The drawing under review shows one solid part. Ordinate dimensions are in mm from its lowest x, y, z. A direction names the side the tool comes from. Coordinates: 2 decimals unless noted, no trailing zeros. Order: outer loops, then holes, each group sorted by start corner. A loop starts at its lowest first (then second) coordinate and runs counter-clockwise, first axis right, second up.
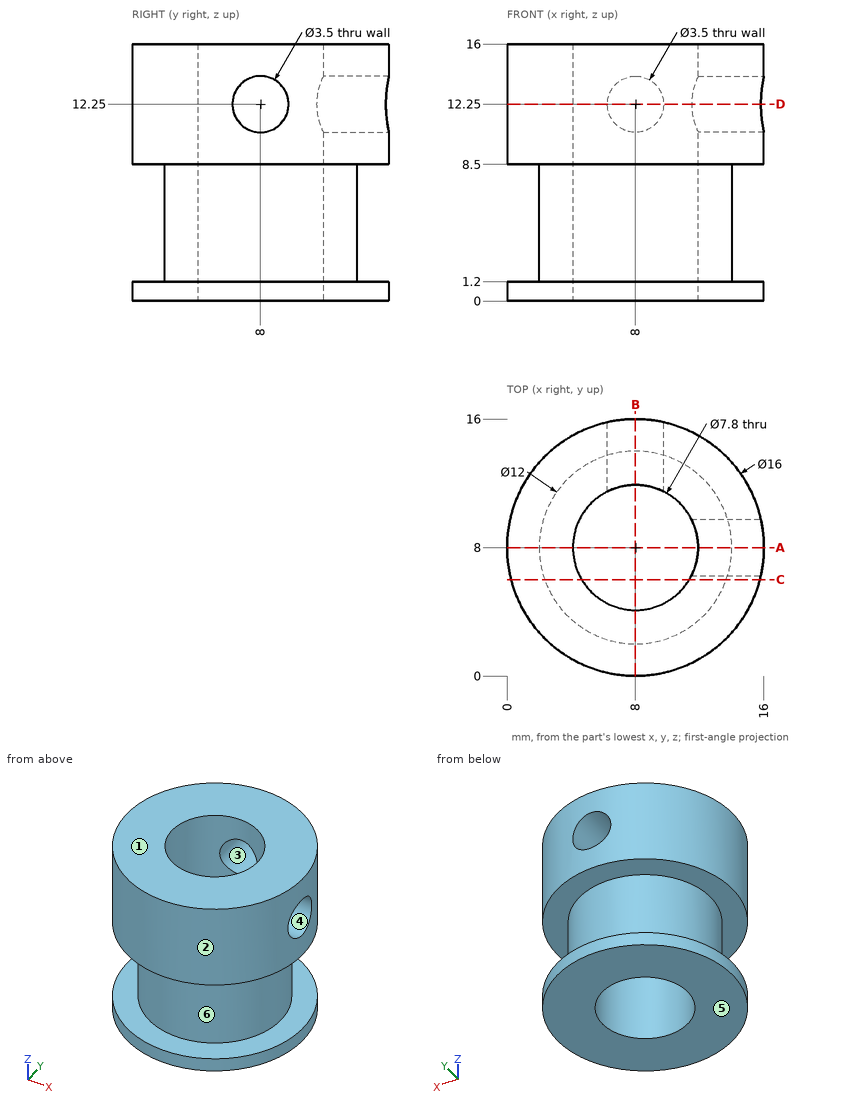
(1) We need section C-C, the plane y = 6. Write out the cut boundary in (x, z).
A:
outline: (0.25, 0) - (4.65, 0) - (4.65, 16) - (0.25, 16) - (0.25, 8.5) - (2.34, 8.5) - (2.34, 1.2) - (0.25, 1.2) - close; (11.35, 0) - (15.75, 0) - (15.75, 1.2) - (13.66, 1.2) - (13.66, 8.5) - (15.75, 8.5) - (15.75, 16) - (11.35, 16) - close
(2) We need section A-A, the plane y = 8. Write out the cut boundary in (x, z), and give its area (4 significant figures).
A:
outline: (0, 0) - (4.1, 0) - (4.1, 16) - (0, 16) - (0, 8.5) - (2, 8.5) - (2, 1.2) - (0, 1.2) - close; (11.9, 0) - (16, 0) - (16, 1.2) - (14, 1.2) - (14, 8.5) - (16, 8.5) - (16, 10.5) - (11.9, 10.5) - close; (11.9, 14) - (16, 14) - (16, 16) - (11.9, 16) - close
area: 87.65 mm2
(3) Machinability: for the marked faces 4, 5 and 6, which of the approach directions +Z, -Z, +X, -X, +Y, -Y give a long, thin tool a straight path to every point of the face, cutting with its end or side? Answer none if there is none.
A:
face 4: +X
face 5: -Z, +X, -X, +Y, -Y
face 6: none
(4) For pin 1 Ø1.5 at (y, z) = (6.5, 11.5) entering from -X; pin 2 Ø4.5 at (x, y) = (8, 8) entering from -Z; pin 3 Ø5 at (y, z) = (2, 7.5) entering from +X; pin 4 Ø1.5 at (y, z) = (4.5, 1.5) entering from +X, all flat-tipped, find the tip position at first contact; note any pin that passes through.
A:
pin 1: stops at x = 0.04
pin 2: passes through
pin 3: stops at x = 15.09
pin 4: stops at x = 15.49
(5) We need section D-D, the plane z = 12.25. Write out the cut boundary in (x, y), and give its area (3 significant figures).
A:
outline: (6.25, 11.49) - (6.25, 15.81) arc R8 ccw (long way) to (15.81, 6.25) - (11.49, 6.25) arc R3.9 cw (long way) to start; (9.75, 11.49) arc R3.9 cw to (11.49, 9.75) - (15.81, 9.75) arc R8 ccw to (9.75, 15.81) - close
area: 124 mm2
(6) Wall thickness on probe 1 along Y at (x, z) = (8, 10); probe 2 along Z at (x, y) = (2, 12.75); probe 3 along Y at (x, z) = (7, 1.5): over which ranges is each line inside the solid? List them lowest first.
A:
probe 1: y = 0 to 4.1, 11.9 to 16
probe 2: z = 0 to 1.2, 8.5 to 16
probe 3: y = 2.08 to 4.23, 11.77 to 13.92
(7) Draft analysis for pull direction X (two halves, no side actions). For the marked faces 1, 2 and 3, state which applies: released by +X, released by -X, zero draft, split by the parting line, or undercut.
A:
face 1: zero draft
face 2: split by the parting line
face 3: undercut
